The listing builds one solid part. Answer for the finished solid, in the listing's coordinates (mm). Coordinates: 2 decimals unless noted, no trailing zeros. Loops run counter-clockwise (first coordinate to the right, second up) from the corner with the lowest first, then second, coordinate; pieces in that order, holes last. Notation, with made-up numbers: M -17,25 L 20,25 A18 cw 20,55 Z; hole C -24,30 d7. An arc over 180 degrees is marked long. Answer as a JSON object with one key per item and string values. Group by question number.
1. Given pin 1 (1.5 mm diameter, centred on y = 106, z = -30.5, fed in from -X); pin 2 (0.6 mm diameter, centred on x = -59, z = -90, fed in from -Y); pin 3 (0.6 mm diameter, centred on x = -58.5, y = 49, fed in from +Z), each flat-ended and moving along its own axis, determine where each tip first touches the part or whether it passes through.
2. A cutting plane is placed at A-A on z = -85. Give the vertices of the cut face in (x, y).
3. A cutting plane is placed at D-D on y = 16. Give the vertices of the cut face in (x, z).
4. A cutting plane is placed at C-C on z = -58. Give the vertices of the cut face in (x, y).
5. Straight lines are drawn through the part: L1, parallel to X at y = 37.5, z = -93; L2, parallel to X at y = 6, z = -107.5. For each, find the intervals that lie inside material, in ascending order.
6. A cutting plane is placed at B-B on y = 105. Give the vertices of the cut face in (x, z), and give its area (3 significant figures).
from build123d import *

# Parameters (mm, degrees)
SKETCH2_W           = 190
SKETCH2_H           = 190
BOSS_EXTRUDE1_DEPTH = 130
SKETCH3_W           = 170
SKETCH3_H           = 110
BOSS_EXTRUDE2_DEPTH = 2
SKETCH4_R           = 4
BOSS_EXTRUDE3_DEPTH = 8


with BuildPart() as part:
    # Sketch2 → Boss-Extrude1 (new body)
    with BuildSketch(Plane(origin=(0, 0, 0), x_dir=(1, 0, 0), z_dir=(0, 1, 0))):
        with Locations((37.344584985, 55)):
            Rectangle(SKETCH2_W, SKETCH2_H)
    extrude(amount=BOSS_EXTRUDE1_DEPTH)

    # Sketch3 → Boss-Extrude2 (add)
    with BuildSketch(Plane.ZY.offset(57.655415015)):
        with Locations((-55, 65)):
            Rectangle(SKETCH3_W, SKETCH3_H)
    extrude(amount=BOSS_EXTRUDE2_DEPTH)

    # Sketch4 → Boss-Extrude3 (add)
    with BuildSketch(Plane.ZY.offset(59.655415015)):
        with Locations((-25, 25)):
            Circle(SKETCH4_R)
        with Locations((-45, 25)):
            Circle(SKETCH4_R)
        with Locations((-25, 105)):
            Circle(SKETCH4_R)
        with Locations((-65, 25)):
            Circle(SKETCH4_R)
        with Locations((-85, 25)):
            Circle(SKETCH4_R)
        with Locations((-45, 105)):
            Circle(SKETCH4_R)
        with Locations((-65, 105)):
            Circle(SKETCH4_R)
        with Locations((-85, 105)):
            Circle(SKETCH4_R)
    extrude(amount=BOSS_EXTRUDE3_DEPTH)


solid = part.part
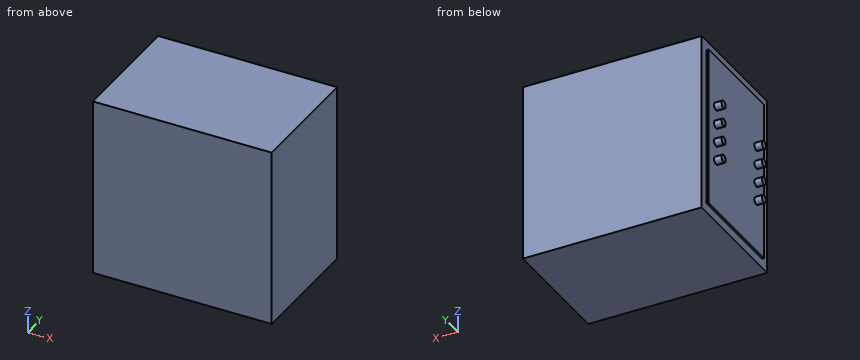
From the geometry:
{
 "1": {"pin 1": "stops at x = -59.66", "pin 2": "stops at y = 10", "pin 3": "stops at z = 30"},
 "2": {"outline": "M -67.66,21 L -59.66,21 L -59.66,10 L -57.66,10 L -57.66,0 L 132.34,0 L 132.34,130 L -57.66,130 L -57.66,120 L -59.66,120 L -59.66,109 L -67.66,109 L -67.66,101 L -59.66,101 L -59.66,29 L -67.66,29 Z"},
 "3": {"outline": "M -59.66,-140 L -57.66,-140 L -57.66,-150 L 132.34,-150 L 132.34,40 L -57.66,40 L -57.66,30 L -59.66,30 Z"},
 "4": {"outline": "M -59.66,10 L -57.66,10 L -57.66,0 L 132.34,0 L 132.34,130 L -57.66,130 L -57.66,120 L -59.66,120 Z"},
 "5": {"L1": "x = -59.66 to 132.34", "L2": "x = -57.66 to 132.34"},
 "6": {"outline": "M -67.66,-89 L -59.66,-89 L -59.66,-140 L -57.66,-140 L -57.66,-150 L 132.34,-150 L 132.34,40 L -57.66,40 L -57.66,30 L -59.66,30 L -59.66,-21 L -67.66,-21 L -67.66,-29 L -59.66,-29 L -59.66,-41 L -67.66,-41 L -67.66,-49 L -59.66,-49 L -59.66,-61 L -67.66,-61 L -67.66,-69 L -59.66,-69 L -59.66,-81 L -67.66,-81 Z", "area": "36,700 mm²"}
}
